from build123d import *

# Parameters (mm, degrees)
SKETCH1_W           = 150
SKETCH1_H           = 200
BOSS_EXTRUDE1_DEPTH = 80
SKETCH2_R           = 3
HOLE_1_DEPTH        = 100
CUT_EXTRUDE2_DEPTH  = 75
FILLET1_R           = 10
BOSS_EXTRUDE2_START = 2
BOSS_EXTRUDE2_DEPTH = 2
SKETCH5_R           = 6
HOLE_2_DEPTH        = 90
SKETCH6_R           = 5
SKETCH6_R_2         = 3
BOSS_EXTRUDE3_DEPTH = 7.5


with BuildPart() as part:
    # Sketch1 → Boss-Extrude1 (new body)
    with BuildSketch(Plane(origin=(0, 0, 0), x_dir=(1, 0, 0), z_dir=(0, 1, 0))):
        with Locations((75, 100)):
            Rectangle(SKETCH1_W, SKETCH1_H)
    extrude(amount=BOSS_EXTRUDE1_DEPTH)

    # Sketch2 → Hole-1 (cut)
    with BuildSketch(Plane(origin=(0, 80, 0), x_dir=(1, 0, 0), z_dir=(0, 1, 0))):
        with Locations(Location((9.5, 190.5, 0), (0, 0, 270))):
            Circle(SKETCH2_R)
        with Locations(Location((140.5, 190.5, 0), (0, 0, 270))):
            Circle(SKETCH2_R)
        with Locations(Location((140.5, 9.5, 0), (0, 0, 270))):
            Circle(SKETCH2_R)
        with Locations(Location((9.5, 9.5, 0), (0, 0, 270))):
            Circle(SKETCH2_R)
    extrude(amount=-HOLE_1_DEPTH, mode=Mode.SUBTRACT)

    # Sketch3 → Cut-Extrude2 (cut)
    with BuildSketch(Plane(origin=(0, 80, 0), x_dir=(1, 0, 0), z_dir=(0, 1, 0))):
        with BuildLine():
            Line((21, 194.973112847), (129, 194.973112847))
            ThreePointArc((129, 194.973112847), (130.414213562, 194.387326409), (131, 192.973112847))
            Line((131, 192.973112847), (131, 189.973112847))
            ThreePointArc((131, 189.973112847), (133.645537903, 183.626537592), (140, 181))
            Line((140, 181), (143, 181))
            ThreePointArc((143, 181), (144.414213562, 180.414213562), (145, 179))
            Line((145, 179), (145, 21))
            ThreePointArc((145, 21), (144.414213562, 19.585786438), (143, 19))
            Line((143, 19), (140, 19))
            ThreePointArc((140, 19), (133.636038969, 16.363961031), (131, 10))
            Line((131, 10), (131, 7))
            ThreePointArc((131, 7), (130.414213562, 5.585786438), (129, 5))
            Line((129, 5), (21, 5))
            ThreePointArc((21, 5), (19.585786438, 5.585786438), (19, 7))
            Line((19, 7), (19, 10))
            ThreePointArc((19, 10), (16.363961031, 16.363961031), (10, 19))
            Line((10, 19), (7, 19))
            ThreePointArc((7, 19), (5.585786438, 19.585786438), (5, 21))
            Line((5, 21), (5, 179))
            ThreePointArc((5, 179), (5.585786438, 180.414213562), (7, 181))
            Line((7, 181), (10, 181))
            ThreePointArc((10, 181), (16.354462097, 183.626537592), (19, 189.973112847))
            Line((19, 189.973112847), (19, 192.973112847))
            ThreePointArc((19, 192.973112847), (19.585786438, 194.387326409), (21, 194.973112847))
        make_face()
    extrude(amount=-CUT_EXTRUDE2_DEPTH, mode=Mode.SUBTRACT)

    # Fillet1
    fillet1_edges = [part.edges().sort_by_distance(p)[0] for p in [
        (0, 40, -200),
        (150, 40, -200),
        (150, 40, 0),
        (0, 40, 0),
    ]]
    fillet(fillet1_edges, radius=FILLET1_R)

    # Sketch4 → Boss-Extrude2 (add)
    with BuildSketch(Plane(origin=(0, 80, 0), x_dir=(1, 0, 0), z_dir=(0, 1, 0)).offset(BOSS_EXTRUDE2_START)):
        with BuildLine():
            Line((4, 179), (4, 21))
            ThreePointArc((4, 21), (4.878679656, 18.878679656), (7, 18))
            Line((7, 18), (10, 18))
            ThreePointArc((10, 18), (15.656854249, 15.656854249), (18, 10))
            Line((18, 10), (18, 7))
            ThreePointArc((18, 7), (18.878679656, 4.878679656), (21, 4))
            Line((21, 4), (129, 4))
            ThreePointArc((129, 4), (131.121320344, 4.878679656), (132, 7))
            Line((132, 7), (132, 10))
            ThreePointArc((132, 10), (134.343145751, 15.656854249), (140, 18))
            Line((140, 18), (143, 18))
            ThreePointArc((143, 18), (145.121320344, 18.878679656), (146, 21))
            Line((146, 21), (146, 179))
            ThreePointArc((146, 179), (145.121320344, 181.121320344), (143, 182))
            Line((143, 182), (139.998459858, 182))
            ThreePointArc((139.998459858, 182), (134.344236882, 184.326302053), (132, 189.973112847))
            Line((132, 189.973112847), (132, 192.973112847))
            ThreePointArc((132, 192.973112847), (131.121320344, 195.09443319), (129, 195.973112847))
            Line((129, 195.973112847), (21, 195.973112847))
            ThreePointArc((21, 195.973112847), (18.878679656, 195.09443319), (18, 192.973112847))
            Line((18, 192.973112847), (18, 189.973112847))
            ThreePointArc((18, 189.973112847), (15.655763118, 184.326302053), (10.001540142, 182))
            Line((10.001540142, 182), (7, 182))
            ThreePointArc((7, 182), (4.878679656, 181.121320344), (4, 179))
        make_face()
        with BuildLine():
            Line((5, 179), (5, 21))
            ThreePointArc((5, 21), (5.585786438, 19.585786438), (7, 19))
            Line((7, 19), (10, 19))
            ThreePointArc((10, 19), (16.363961031, 16.363961031), (19, 10))
            Line((19, 10), (19, 7))
            ThreePointArc((19, 7), (19.585786438, 5.585786438), (21, 5))
            Line((21, 5), (129, 5))
            ThreePointArc((129, 5), (130.414213562, 5.585786438), (131, 7))
            Line((131, 7), (131, 10))
            ThreePointArc((131, 10), (133.636038969, 16.363961031), (140, 19))
            Line((140, 19), (143, 19))
            ThreePointArc((143, 19), (144.414213562, 19.585786438), (145, 21))
            Line((145, 21), (145, 179))
            ThreePointArc((145, 179), (144.414213562, 180.414213562), (143, 181))
            Line((143, 181), (140, 181))
            ThreePointArc((140, 181), (133.637674623, 183.61865075), (131, 189.973112847))
            Line((131, 189.973112847), (131, 192.973112847))
            ThreePointArc((131, 192.973112847), (130.414213562, 194.387326409), (129, 194.973112847))
            Line((129, 194.973112847), (21, 194.973112847))
            ThreePointArc((21, 194.973112847), (19.585786438, 194.387326409), (19, 192.973112847))
            Line((19, 192.973112847), (19, 189.973112847))
            ThreePointArc((19, 189.973112847), (16.362325377, 183.61865075), (10, 181))
            Line((10, 181), (7, 181))
            ThreePointArc((7, 181), (5.585786438, 180.414213562), (5, 179))
        make_face(mode=Mode.SUBTRACT)
    extrude(amount=-BOSS_EXTRUDE2_DEPTH)

    # Sketch5 → Hole-2 (cut)
    with BuildSketch(Plane(origin=(0, 80, 0), x_dir=(1, 0, 0), z_dir=(0, 1, 0))):
        with Locations(Location((9.5, 9.5, 0), (0, 0, 270))):
            Circle(SKETCH5_R)
        with Locations(Location((140.5, 9.5, 0), (0, 0, 270))):
            Circle(SKETCH5_R)
        with Locations(Location((140.5, 190.5, 0), (0, 0, 270))):
            Circle(SKETCH5_R)
        with Locations(Location((9.5, 190.5, 0), (0, 0, 270))):
            Circle(SKETCH5_R)
    extrude(amount=-HOLE_2_DEPTH, mode=Mode.SUBTRACT)

    # Sketch6 → Boss-Extrude3 (add)
    # profile 1 of 12: a face of its own
    with BuildSketch(Plane(origin=(0, 5, 0), x_dir=(1, 0, 0), z_dir=(0, 1, 0))):
        with Locations(Location((130, 100, 0), (0, 0, 90))):
            Circle(SKETCH6_R)
        with Locations(Location((130, 100, 0), (0, 0, 270))):
            Circle(SKETCH6_R_2, mode=Mode.SUBTRACT)
    # profile 2 of 12: a face of its own
    with BuildSketch(Plane(origin=(0, 5, 0), x_dir=(1, 0, 0), z_dir=(0, 1, 0))):
        with Locations(Location((130, 140, 0), (0, 0, 90))):
            Circle(SKETCH6_R)
        with Locations(Location((130, 140, 0), (0, 0, 270))):
            Circle(SKETCH6_R_2, mode=Mode.SUBTRACT)
    # profile 3 of 12: a face of its own
    with BuildSketch(Plane(origin=(0, 5, 0), x_dir=(1, 0, 0), z_dir=(0, 1, 0))):
        with Locations(Location((115, 179.973112847, 0), (0, 0, 90))):
            Circle(SKETCH6_R)
        with Locations(Location((115, 179.973112847, 0), (0, 0, 270))):
            Circle(SKETCH6_R_2, mode=Mode.SUBTRACT)
    # profile 4 of 12: a face of its own
    with BuildSketch(Plane(origin=(0, 5, 0), x_dir=(1, 0, 0), z_dir=(0, 1, 0))):
        with Locations(Location((35, 179.973112847, 0), (0, 0, 90))):
            Circle(SKETCH6_R)
        with Locations(Location((35, 179.973112847, 0), (0, 0, 90))):
            Circle(SKETCH6_R_2, mode=Mode.SUBTRACT)
    # profile 5 of 12: a face of its own
    with BuildSketch(Plane(origin=(0, 5, 0), x_dir=(1, 0, 0), z_dir=(0, 1, 0))):
        with Locations(Location((20, 140, 0), (0, 0, 90))):
            Circle(SKETCH6_R)
        with Locations(Location((20, 140, 0), (0, 0, 90))):
            Circle(SKETCH6_R_2, mode=Mode.SUBTRACT)
    # profile 6 of 12: a face of its own
    with BuildSketch(Plane(origin=(0, 5, 0), x_dir=(1, 0, 0), z_dir=(0, 1, 0))):
        with Locations(Location((20, 100, 0), (0, 0, 90))):
            Circle(SKETCH6_R)
        with Locations(Location((20, 100, 0), (0, 0, 90))):
            Circle(SKETCH6_R_2, mode=Mode.SUBTRACT)
    # profile 7 of 12: a face of its own
    with BuildSketch(Plane(origin=(0, 5, 0), x_dir=(1, 0, 0), z_dir=(0, 1, 0))):
        with Locations(Location((75, 182.973112847, 0), (0, 0, 90))):
            Circle(SKETCH6_R)
        with Locations(Location((75, 182.973112847, 0), (0, 0, 270))):
            Circle(SKETCH6_R_2, mode=Mode.SUBTRACT)
    # profile 8 of 12: a face of its own
    with BuildSketch(Plane(origin=(0, 5, 0), x_dir=(1, 0, 0), z_dir=(0, 1, 0))):
        with Locations(Location((75, 17.026887153, 0), (0, 0, 90))):
            Circle(SKETCH6_R)
        with Locations(Location((75, 17.026887153, 0), (0, 0, 90))):
            Circle(SKETCH6_R_2, mode=Mode.SUBTRACT)
    # profile 9 of 12: a face of its own
    with BuildSketch(Plane(origin=(0, 5, 0), x_dir=(1, 0, 0), z_dir=(0, 1, 0))):
        with Locations(Location((20, 60, 0), (0, 0, 90))):
            Circle(SKETCH6_R)
        with Locations(Location((20, 60, 0), (0, 0, 270))):
            Circle(SKETCH6_R_2, mode=Mode.SUBTRACT)
    # profile 10 of 12: a face of its own
    with BuildSketch(Plane(origin=(0, 5, 0), x_dir=(1, 0, 0), z_dir=(0, 1, 0))):
        with Locations(Location((35, 20.026887153, 0), (0, 0, 90))):
            Circle(SKETCH6_R)
        with Locations(Location((35, 20.026887153, 0), (0, 0, 270))):
            Circle(SKETCH6_R_2, mode=Mode.SUBTRACT)
    # profile 11 of 12: a face of its own
    with BuildSketch(Plane(origin=(0, 5, 0), x_dir=(1, 0, 0), z_dir=(0, 1, 0))):
        with Locations(Location((115, 20.026887153, 0), (0, 0, 90))):
            Circle(SKETCH6_R)
        with Locations(Location((115, 20.026887153, 0), (0, 0, 90))):
            Circle(SKETCH6_R_2, mode=Mode.SUBTRACT)
    # profile 12 of 12: a face of its own
    with BuildSketch(Plane(origin=(0, 5, 0), x_dir=(1, 0, 0), z_dir=(0, 1, 0))):
        with Locations(Location((130, 60, 0), (0, 0, 90))):
            Circle(SKETCH6_R)
        with Locations(Location((130, 60, 0), (0, 0, 90))):
            Circle(SKETCH6_R_2, mode=Mode.SUBTRACT)
    extrude(amount=BOSS_EXTRUDE3_DEPTH)


solid = part.part
Read the model definition and answer for the solid it produces. Units are mm, in the model's axes. Coordinates: 2 decimals unless noted, no trailing zeros. Loops run counter-clockwise (first coordinate to the right, second up) from the corner with the lowest first, then second, coordinate; pieces in that order, holes last. Notation, with made-up numbers: (-7.5, -35.75) -> (40.5, -35.75) arc R18 ccw to (40.5, -8.75) -> close; hole circle Ø10 at (69, 5.25). An arc over 180 degrees is marked (long way). Write item = value, one per line. Start each with the question number.
1) The part is cut by section A-A, the plane z = -31.5. Determine the outline of the cut face in (x, y), plus the area to 3 significant figures.
2) The part is cut by section B-B, the plane y = 9. State how many separate pieces and enclosed holes the cut face has, plus the area to 3 significant figures.
3) Find the intervals of material crossed by L1, parallel to X at y = 54, z = -9; L2, parallel to X at y = 9, z = -100; L3, parallel to X at y = 35, z = -9.5, in increasing order. Write a range as from..to.
4) Given P1, Ø0.6, axis at x = 83, y = 81.5, coming from the -Z side; P2, Ø1.5, axis at x = 8, y = 56.5, coming from the +Z side; P3, Ø1.5, axis at y = 55.5, z = -9, coming from the -X side, each flat-ended and moving along its own axis, determine where each tip first touches the part or whether it passes through.
5) The part is cut by section C-C, the plane x = 75. Determine the outline of the cut face in (y, z).
6) The mould has two halves that part along X. Classify faces 1 (the face through (2.85, 40.56, -3.01)), 2 (the face through (38.3, 12.5, -20)): pulls with the +X half, pulls with the -X half, needs draft (parallel to the pull), parting line crosses it, or undercut.
Result:
q1.outline = (0, 0) -> (150, 0) -> (150, 80) -> (146, 80) -> (146, 82) -> (145, 82) -> (145, 5) -> (5, 5) -> (5, 82) -> (4, 82) -> (4, 80) -> (0, 80) -> close
q1.area = 1,500 mm²
q2.separate_pieces = 13
q2.enclosed_holes = 17
q2.area = 4,190 mm²
q3.L1 = 0.05..3.52, 15.48..19, 131..134.52, 146.48..149.95
q3.L2 = 0..5, 15..17, 23..25, 125..127, 133..135, 145..150
q3.L3 = 0.01..3.5, 15.5..19, 131..134.5, 146.5..149.99
q4.P1 = -195.97
q4.P2 = -0.08
q4.P3 = 0
q5.outline = (0, -200) -> (80, -200) -> (80, -195.97) -> (82, -195.97) -> (82, -194.97) -> (5, -194.97) -> (5, -187.97) -> (12.5, -187.97) -> (12.5, -185.97) -> (5, -185.97) -> (5, -179.97) -> (12.5, -179.97) -> (12.5, -177.97) -> (5, -177.97) -> (5, -22.03) -> (12.5, -22.03) -> (12.5, -20.03) -> (5, -20.03) -> (5, -14.03) -> (12.5, -14.03) -> (12.5, -12.03) -> (5, -12.03) -> (5, -5) -> (82, -5) -> (82, -4) -> (80, -4) -> (80, 0) -> (0, 0) -> close
q6.face_1 = pulls with the -X half
q6.face_2 = undercut
